Input: dimensioned drawing with shaded views. Units: mm. Origin: part minimum x, y, z. Round coordinates to 2 decimals unless told otherwise and drop trailing zeros. Order: outer loops, then holes, each group sorted by start corner. A loop starts at its lowest first (then second) coordinate and runs counter-clockwise, first axis right, second up. Notation, with made-up numbers: M 83.5,13.5 L 99.5,13.5 A25 cw 99.5,47.5 Z; hole C -17,-20 d6. An arc over 180 degrees is marked long. Use one line per item in the form item = value. Start each with the question number.
Q1. Material intervals for probe 1 along Y at (x, z) = (11, 1.5); probe 2 along X at (y, z) = (14.5, 5.25) (1 decimal); probe 3 along Y at (x, z) = (10.75, 4), sorted ascending.
Q2. Pull-direction query (X, two-part tool) for the marked faces 1, 2 and 3; classes: pulls with the +X half, pulls with the -X half, needs draft (parallel to the pull), parting line crosses it, or undercut.
Q3. Section A-A (x = 9.85). Return the cut outline in (y, z).
Q4. Section B-B (y = 14.5). Return the cut outline in (x, z).
Q5. Contact query for flat-ended pins moving along their axis: pin 1 (4 mm diameter, centred on x = 16.5, z = 6.5, fed in from -Y); pin 2 (4 mm diameter, centred on y = 17, z = 7, fed in from +X); pin 3 (4 mm diameter, centred on y = 11.5, z = 2, fed in from -X). Output: stop coordinate, or through.
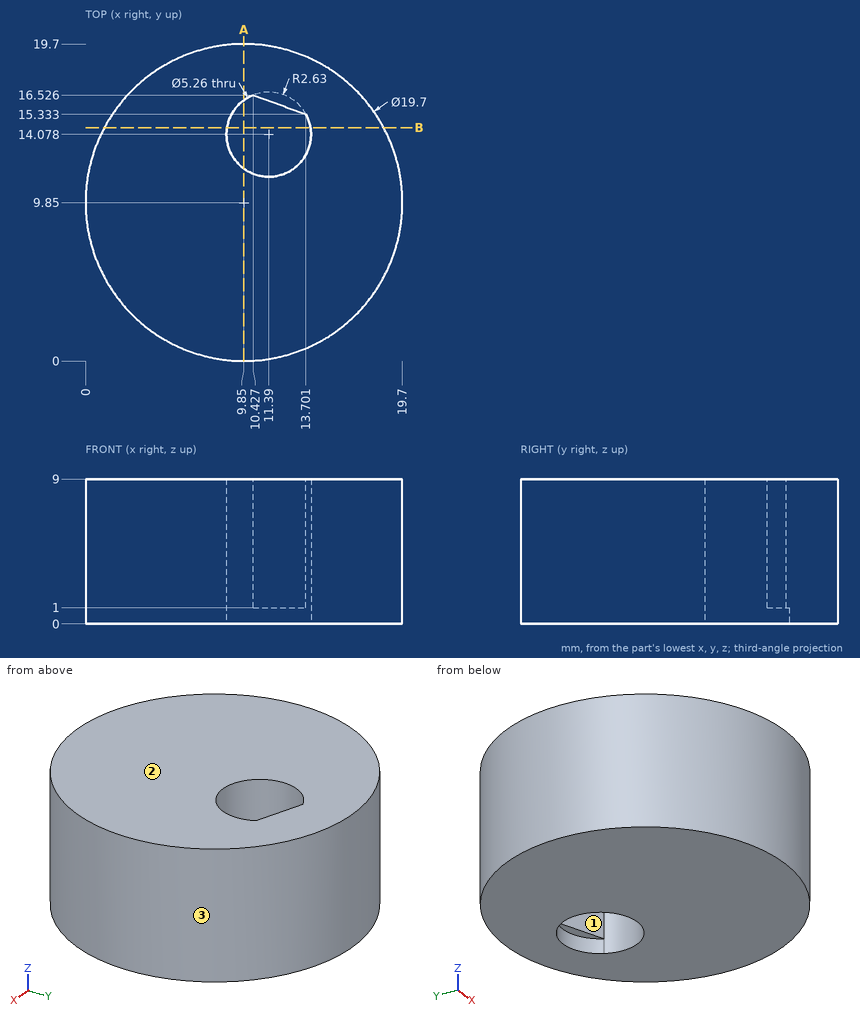
Results list:
q1.probe_1 = 0.07 to 11.48, 16.32 to 19.63
q1.probe_2 = 1.2 to 8.8, 14 to 18.5
q1.probe_3 = 0.04 to 11.53, 16.41 to 19.66
q2.face_1 = undercut
q2.face_2 = needs draft
q2.face_3 = parting line crosses it
q3.outline = M 0,0 L 11.95,0 L 11.95,9 L 0,9 Z; M 16.21,0 L 19.7,0 L 19.7,9 L 16.21,9 Z
q4.outline = M 1.17,0 L 8.79,0 L 8.79,9 L 1.17,9 Z; M 13.99,0 L 18.53,0 L 18.53,9 L 13.99,9 Z
q5.pin_1 = 1.17
q5.pin_2 = 18.25
q5.pin_3 = 0
